Design review of the part built by this model. Coordinates are the model's own, in mm. Give positions to 0.01 mm unless a question says otherwise; leave off trailing zeros. One line per item, written item: value. Start each with the question number.
1) For pin 1 (1.2 mm diameter, centred on y = 40.5, z = 3, fed in from +X); pin 2 (1.1 mm diameter, centred on x = 14, y = -92, fed in from -Z); pin 3 (1.7 mm diameter, centred on x = 2.5, y = -4.5, fed in from +Z), all flat-tipped, find the tip position at first contact; note any pin that passes through.
2) Consider section A-A (y = -59). State how many separate pieces and enclosed holes the cut face has, plus the area to 3 significant figures.
3) Wall thickness on line 1 along Z through (x, y) = (-4.5, -200.5); line 2 along Z through (x, y) = (-11.75, -207.5); line 3 along Z through (x, y) = (2.25, 122): over which ranges is each line inside the solid? List them lowest first. Write a range as from..to.
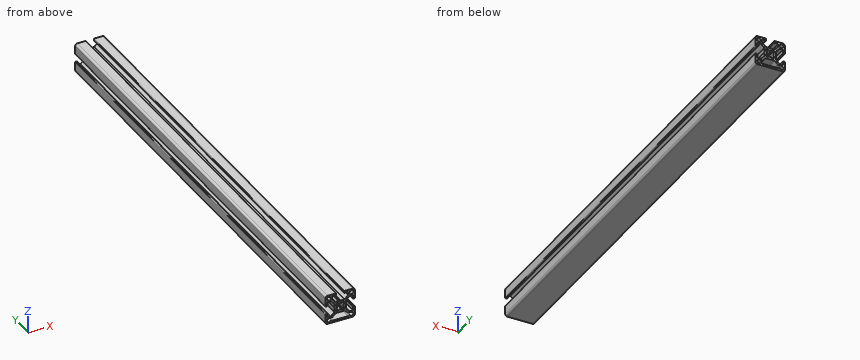
from build123d import *

# Parameters (mm, degrees)
F2_DEPTH = 240


# Not quite as in the source:
# - ends of sketch curves that miss each other by under 0.0002 mm in the source are joined


with BuildPart() as f2:
    # F1 (on Front) → F2 (new body, symmetric)
    with BuildSketch(Plane.XZ):
        with BuildLine():
            Line((8.249944, 9.6642), (4.58573, 5.999986))
            Line((4.58573, 5.999986), (0.653534, 5.999986))
            ThreePointArc((0.653534, 5.999986), (0.5241245494, 5.9829489324), (0.4035341291, 5.9329987764))
            Line((0.4035341291, 5.9329987764), (-5.6e-05, 5.699986))
            Line((-5.6e-05, 5.699986), (-0.403646, 5.932999))
            ThreePointArc((-0.403646, 5.932999), (-0.653646, 5.999986), (-0.9036458709, 5.9329987764))
            Line((-0.9036458709, 5.9329987764), (-1.218942, 5.750963))
            Line((-1.218942, 5.750963), (-2.500056, 5.999986))
            Line((-2.500056, 5.999986), (-4.585842, 5.999986))
            Line((-4.585842, 5.999986), (-8.250056, 9.6642))
            Line((-8.250056, 9.6642), (-8.250056, 12.999986))
            Line((-8.250056, 12.999986), (-4.300056, 12.999986))
            ThreePointArc((-4.300056, 12.999986), (-4.0879239656, 13.0878539656), (-4.000056, 13.299986))
            Line((-4.000056, 13.299986), (-4.000056, 14.699986))
            ThreePointArc((-4.000056, 14.699986), (-4.0879239656, 14.9121180344), (-4.300056, 14.999986))
            Line((-4.300056, 14.999986), (-13.000056, 14.999986))
            ThreePointArc((-13.000056, 14.999986), (-14.4142695624, 14.4141995624), (-15.000056, 12.999986))
            Line((-15.000056, 12.999986), (-15.000056, 4.299986))
            ThreePointArc((-15.000056, 4.299986), (-14.9121880344, 4.0878539656), (-14.700056, 3.999986))
            Line((-14.700056, 3.999986), (-13.300056, 3.999986))
            ThreePointArc((-13.300056, 3.999986), (-13.0879239656, 4.0878539656), (-13.000056, 4.299986))
            Line((-13.000056, 4.299986), (-13.000056, 8.249986))
            Line((-13.000056, 8.249986), (-9.66427, 8.249986))
            Line((-9.66427, 8.249986), (-6.000056, 4.585772))
            Line((-6.000056, 4.585772), (-6.000056, 0.653576))
            ThreePointArc((-6.000056, 0.653576), (-5.9830189324, 0.5241665494), (-5.9330687764, 0.4035761291))
            Line((-5.9330687764, 0.4035761291), (-5.700056, -1.4e-05))
            Line((-5.700056, -1.4e-05), (-5.933069, -0.403604))
            ThreePointArc((-5.933069, -0.403604), (-6.000056, -0.653604), (-5.9330687764, -0.9036038709))
            Line((-5.9330687764, -0.9036038709), (-5.751033, -1.2189))
            Line((-5.751033, -1.2189), (-6.000056, -2.500014))
            Line((-6.000056, -2.500014), (-6.000056, -4.5858))
            Line((-6.000056, -4.5858), (-9.66427, -8.250014))
            Line((-9.66427, -8.250014), (-13.000056, -8.250014))
            Line((-13.000056, -8.250014), (-13.000056, -4.300014))
            ThreePointArc((-13.000056, -4.300014), (-13.0879239656, -4.0878819656), (-13.300056, -4.000014))
            Line((-13.300056, -4.000014), (-14.700056, -4.000014))
            ThreePointArc((-14.700056, -4.000014), (-14.9121880344, -4.0878819656), (-15.000056, -4.300014))
            Line((-15.000056, -4.300014), (-15.000056, -13.000014))
            ThreePointArc((-15.000056, -13.000014), (-14.4142695624, -14.4142275624), (-13.000056, -15.000014))
            Line((-13.000056, -15.000014), (12.999944, -15.000014))
            ThreePointArc((12.999944, -15.000014), (14.4141575624, -14.4142275624), (14.999944, -13.000014))
            Line((14.999944, -13.000014), (14.999944, -4.300014))
            ThreePointArc((14.999944, -4.300014), (14.9120760344, -4.0878819656), (14.699944, -4.000014))
            Line((14.699944, -4.000014), (13.299944, -4.000014))
            ThreePointArc((13.299944, -4.000014), (13.0878119656, -4.0878819656), (12.999944, -4.300014))
            Line((12.999944, -4.300014), (12.999944, -8.250014))
            Line((12.999944, -8.250014), (9.664158, -8.250014))
            Line((9.664158, -8.250014), (5.999944, -4.5858))
            Line((5.999944, -4.5858), (5.999944, -0.653604))
            ThreePointArc((5.999944, -0.653604), (5.9829069324, -0.5241945494), (5.9329567764, -0.4036041291))
            Line((5.9329567764, -0.4036041291), (5.699944, -1.4e-05))
            Line((5.699944, -1.4e-05), (5.932957, 0.403576))
            ThreePointArc((5.932957, 0.403576), (5.999944, 0.653576), (5.9329567764, 0.9035758709))
            Line((5.9329567764, 0.9035758709), (5.750921, 1.218872))
            Line((5.750921, 1.218872), (5.999944, 2.499986))
            Line((5.999944, 2.499986), (5.999944, 4.585772))
            Line((5.999944, 4.585772), (9.664158, 8.249986))
            Line((9.664158, 8.249986), (12.999944, 8.249986))
            Line((12.999944, 8.249986), (12.999944, 4.299986))
            ThreePointArc((12.999944, 4.299986), (13.0878119656, 4.0878539656), (13.299944, 3.999986))
            Line((13.299944, 3.999986), (14.699944, 3.999986))
            ThreePointArc((14.699944, 3.999986), (14.9120760344, 4.0878539656), (14.999944, 4.299986))
            Line((14.999944, 4.299986), (14.999944, 12.999986))
            ThreePointArc((14.999944, 12.999986), (14.4141575624, 14.4141995624), (12.999944, 14.999986))
            Line((12.999944, 14.999986), (4.299944, 14.999986))
            ThreePointArc((4.299944, 14.999986), (4.0878119656, 14.9121180344), (3.999944, 14.699986))
            Line((3.999944, 14.699986), (3.999944, 13.299986))
            ThreePointArc((3.999944, 13.299986), (4.0878119656, 13.0878539656), (4.299944, 12.999986))
            Line((4.299944, 12.999986), (8.249944, 12.999986))
            Line((8.249944, 12.999986), (8.249944, 9.6642))
        make_face()
        with BuildLine():
            Line((-4.171629, -6.000014), (4.171517, -6.000014))
            ThreePointArc((4.171517, -6.000014), (4.5542004324, -6.0761344675), (4.8786237812, -6.2929072188))
            Line((4.8786237812, -6.2929072188), (7.742837, -9.157121))
            ThreePointArc((7.742837, -9.157121), (8.0672605676, -9.3738935325), (8.449944, -9.450014))
            Line((8.449944, -9.450014), (11.073348, -9.450014))
            Line((11.073348, -9.450014), (12.349782, -9.914598))
            ThreePointArc((12.349782, -9.914598), (13.2040603505, -12.8608903949), (10.1374570291, -12.7810479799))
            ThreePointArc((10.1374570291, -12.7810479799), (9.3136995047, -12.3500149751), (8.4911490608, -12.7833470418))
            ThreePointArc((8.4911490608, -12.7833470418), (8.3119125635, -12.9425444809), (8.079175, -13.000014))
            Line((8.079175, -13.000014), (-8.079287, -13.000014))
            ThreePointArc((-8.079287, -13.000014), (-8.3120245635, -12.9425444809), (-8.4912608636, -12.7833469062))
            ThreePointArc((-8.4912608636, -12.7833469062), (-9.3138115047, -12.3500149751), (-10.1375690315, -12.7810479782))
            ThreePointArc((-10.1375690315, -12.7810479782), (-13.2041723505, -12.8608903949), (-12.3498940253, -9.9145979306))
            Line((-12.3498940253, -9.9145979306), (-11.07346, -9.450014))
            Line((-11.07346, -9.450014), (-8.450056, -9.450014))
            ThreePointArc((-8.450056, -9.450014), (-8.0673725676, -9.3738935325), (-7.7429492188, -9.1571207812))
            Line((-7.7429492188, -9.1571207812), (-4.878736, -6.292907))
            ThreePointArc((-4.878736, -6.292907), (-4.5543124324, -6.0761344675), (-4.171629, -6.000014))
        make_face(mode=Mode.SUBTRACT)
        with BuildLine():
            ThreePointArc((-12.3498940253, 9.9145699306), (-13.0435588843, 13.0434888843), (-9.9146399306, 12.3498240253))
            Line((-9.9146399306, 12.3498240253), (-9.547908, 11.342236))
            ThreePointArc((-9.547908, 11.342236), (-9.8735275063, 9.8734575063), (-11.3423061215, 9.5478376661))
            Line((-11.3423061215, 9.5478376661), (-12.3498940253, 9.9145699306))
        make_face(mode=Mode.SUBTRACT)
        with BuildLine():
            ThreePointArc((0.9882629956, -3.2532009855), (-5.6e-05, -3.400014), (-0.9883749956, -3.2532009855))
            ThreePointArc((-0.9883749956, -3.2532009855), (-1.3178396431, -3.2974811593), (-1.5000564258, -3.5755229349))
            ThreePointArc((-1.5000564258, -3.5755229349), (-1.6685571025, -3.8793255231), (-1.994322, -4.000014))
            Line((-1.994322, -4.000014), (-3.500056, -4.000014))
            ThreePointArc((-3.500056, -4.000014), (-3.8536093906, -3.8535673906), (-4.000056, -3.500014))
            Line((-4.000056, -3.500014), (-4.000056, -1.99428))
            ThreePointArc((-4.000056, -1.99428), (-3.8793675231, -1.6685151025), (-3.5755649263, -1.5000144822))
            ThreePointArc((-3.5755649263, -1.5000144822), (-3.2975231593, -1.3177976431), (-3.2532441585, -0.9883290481))
            ThreePointArc((-3.2532441585, -0.9883290481), (-3.400056, -1.4e-05), (-3.2532429855, 0.9883049956))
            ThreePointArc((-3.2532429855, 0.9883049956), (-3.2975231593, 1.3177696431), (-3.5755649349, 1.4999864258))
            ThreePointArc((-3.5755649349, 1.4999864258), (-3.8793675231, 1.6684871025), (-4.000056, 1.994252))
            Line((-4.000056, 1.994252), (-4.000056, 3.499986))
            ThreePointArc((-4.000056, 3.499986), (-3.8536093906, 3.8535393906), (-3.500056, 3.999986))
            Line((-3.500056, 3.999986), (-1.994322, 3.999986))
            ThreePointArc((-1.994322, 3.999986), (-1.6685571025, 3.8792975231), (-1.5000564822, 3.5754949263))
            ThreePointArc((-1.5000564822, 3.5754949263), (-1.3178396431, 3.2974531593), (-0.9883710481, 3.2531741585))
            ThreePointArc((-0.9883710481, 3.2531741585), (-5.6e-05, 3.399986), (0.9882629956, 3.2531729855))
            ThreePointArc((0.9882629956, 3.2531729855), (1.3177276431, 3.2974531593), (1.4999444258, 3.5754949349))
            ThreePointArc((1.4999444258, 3.5754949349), (1.6684451025, 3.8792975231), (1.99421, 3.999986))
            Line((1.99421, 3.999986), (3.499944, 3.999986))
            ThreePointArc((3.499944, 3.999986), (3.8534973906, 3.8535393906), (3.999944, 3.499986))
            Line((3.999944, 3.499986), (3.999944, 1.994252))
            ThreePointArc((3.999944, 1.994252), (3.8792555231, 1.6684871025), (3.5754529263, 1.4999864822))
            ThreePointArc((3.5754529263, 1.4999864822), (3.2974111593, 1.3177696431), (3.2531321585, 0.9883010481))
            ThreePointArc((3.2531321585, 0.9883010481), (3.399944, -1.4e-05), (3.2531309855, -0.9883329956))
            ThreePointArc((3.2531309855, -0.9883329956), (3.2974111593, -1.3177976431), (3.5754529349, -1.5000144258))
            ThreePointArc((3.5754529349, -1.5000144258), (3.8792555231, -1.6685151025), (3.999944, -1.99428))
            Line((3.999944, -1.99428), (3.999944, -3.500014))
            ThreePointArc((3.999944, -3.500014), (3.8534973906, -3.8535673906), (3.499944, -4.000014))
            Line((3.499944, -4.000014), (1.99421, -4.000014))
            ThreePointArc((1.99421, -4.000014), (1.6684451025, -3.8793255231), (1.4999444822, -3.5755229263))
            ThreePointArc((1.4999444822, -3.5755229263), (1.3177276431, -3.2974811593), (0.9882629956, -3.2532009855))
        make_face(mode=Mode.SUBTRACT)
        with BuildLine():
            ThreePointArc((11.3421941215, 9.5478376661), (9.8734155063, 9.8734575063), (9.5477956661, 11.3422361215))
            Line((9.5477956661, 11.3422361215), (9.914528, 12.349824))
            ThreePointArc((9.914528, 12.349824), (13.0434468843, 13.0434888843), (12.3497820253, 9.9145699306))
            Line((12.3497820253, 9.9145699306), (11.3421941215, 9.5478376661))
        make_face(mode=Mode.SUBTRACT)
    extrude(amount=F2_DEPTH, both=True)


solid = f2.part
Checked values:
1. pin 1: stops at x = 6
1. pin 2: stops at z = -14.95
1. pin 3: stops at z = 6
2. separate pieces: 1
2. enclosed holes: 4
2. area: 322 mm^2
3. line 1: z = -15..-13, -6.06..6, 13..15
3. line 2: z = -15..-13.6, -9.7..-8.25, 8.25..9.7, 13.6..15
3. line 3: z = -15..-13, -6..-4, 4..6
